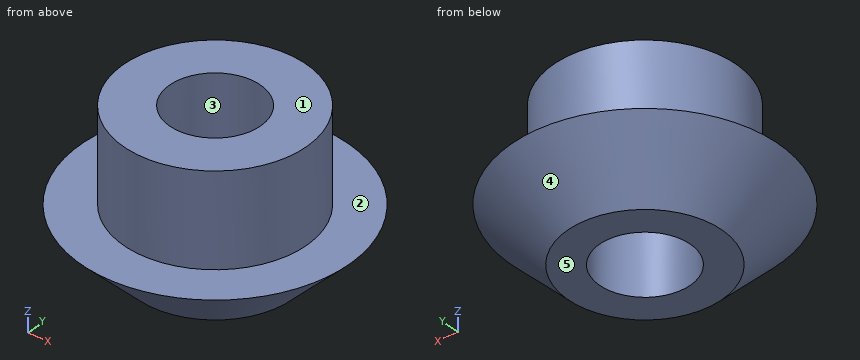
from build123d import *

# Parameters (mm, degrees)
ESQUISSE1_R        = 6.22
ESQUISSE1_R_2      = 3.095
BOSS_EXTRU_1_DEPTH = 10.14
ESQUISSE2_R        = 9.1
ESQUISSE2_R_2      = 6.22
BOSS_EXTRU_2_DEPTH = 3.85


# Read off the part's stored shape, not the designer's step: Enl_vement de mati_re-Balayage1
with BuildPart() as part:
    # Esquisse1 → Boss.-Extru.1 (new body)
    with BuildSketch(Plane.XY):
        Circle(ESQUISSE1_R)
        Circle(ESQUISSE1_R_2, mode=Mode.SUBTRACT)
    extrude(amount=BOSS_EXTRU_1_DEPTH)

    # Esquisse2 → Boss.-Extru.2 (add)
    with BuildSketch(Plane(origin=(0, 0, 0), x_dir=(-1, 0, 0), z_dir=(0, 0, -1))):
        Circle(ESQUISSE2_R)
        Circle(ESQUISSE2_R_2, mode=Mode.SUBTRACT)
    extrude(amount=-BOSS_EXTRU_2_DEPTH)

    # Enl_vement de mati_re-Balayage1 outline → Enl_vement de mati_re-Balayage1 (revolve, cut)
    with BuildSketch(Plane.XZ):
        Polygon((9.1, 3.85), (5.25, 0), (9.1, 0), align=None)
    revolve(axis=Axis((0, 0, 0), (0, 0, 1)), mode=Mode.SUBTRACT)


solid = part.part
Here's how the part is built. I have some questions about the finished solid (model axes, mm). Face numbers are marked on the shaded views. A direction names the side the tool comes from. Coordinates: 2 decimals unless noted, no trailing zeros. Loops run counter-clockwise (first coordinate to the right, second up) from the corner with the lowest first, then second, coordinate; pieces in that order, holes last.
1. For the marked faces 1 and 2, which set-ups out of +Z, -Z, +X, -X, +Y, -Y let a thin tool reach every point of the face, with its end or its side?
2. Imagine slicing it at C-C, the plane z = 3.25. Please give me the cut outline in (x, y) (3 decimals).
3. For P1, Ø2, axis at x = 5, z = 4.5, coming from the +Y side; P2, Ø5, axis at y = -7, z = 2, coming from the +X side; P3, Ø5, axis at y = 3, z = 8.5, coming from the -X side, each with a flat end and sliding along its axis, tell me the tip position at first contact or that it passes through.
4. I need wall thicknesses on L1, parallel to Y at x = 0, z = 4.75 (3 decimals); L2, parallel to Y at x = -0.75, z = 4.5; L3, parallel to X at y = 2, z = 8.5. Which ranges of each line are inside material? Lowest first, please.
5. Imagine slicing it at A-A, the plane y = 0. Please give me the cut outline in (x, z) (3 decimals).
6. Imagine slicing it at D-D, the plane z = 4.75. Please give me the cut outline in (x, y) (3 decimals).
7. If we mould it in two halves opening along X, with no side actions, what happens to the marked faces 3, 4 and 5? For each: pulls with the +X half, pulls with the -X half, needs draft (parallel to the pull), parting line crosses it, or undercut.
Taken from the geometry:
1. face 1: +Z, +X, -X, +Y, -Y
1. face 2: +Z
2. outline: circle Ø17 at (0, 0); hole circle Ø6.19 at (0, 0)
3. P1: stops at y = 8.05
3. P2: stops at x = 7.38
3. P3: stops at x = -6.2
4. L1: y = -6.22 to -3.095, 3.095 to 6.22
4. L2: y = -6.17 to -3, 3 to 6.17
4. L3: x = -5.89 to -2.36, 2.36 to 5.89
5. outline: (-9.1, 3.85) - (-5.25, 0) - (-3.095, 0) - (-3.095, 10.14) - (-6.22, 10.14) - (-6.22, 3.85) - close; (3.095, 0) - (5.25, 0) - (9.1, 3.85) - (6.22, 3.85) - (6.22, 10.14) - (3.095, 10.14) - close
6. outline: circle Ø12.44 at (0, 0); hole circle Ø6.19 at (0, 0)
7. face 3: undercut
7. face 4: parting line crosses it
7. face 5: needs draft
